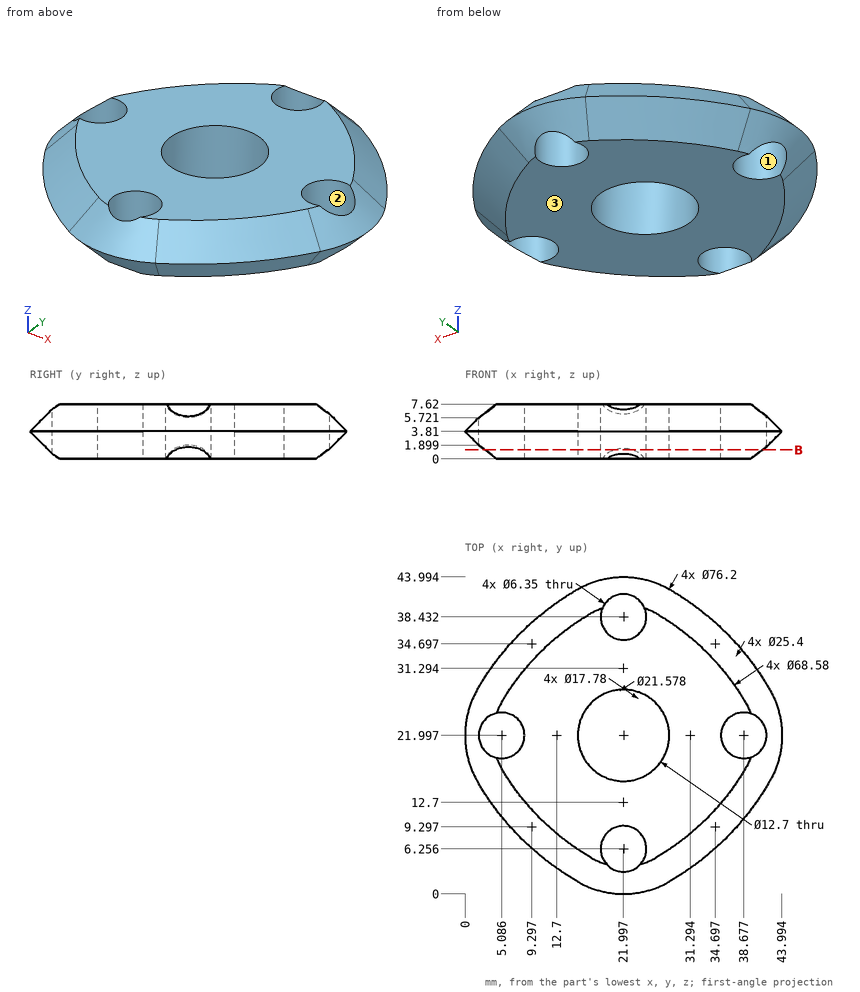
Geometry check sheet. Reference: drawing and pictorial views, mm from the part's lowest x, y, z. Give positions to 0.01 mm unless a question says otherwise; leave off trailing zeros.
1. Go/stop test with flat-tipped pins: pin 1 Ø3 at (y, z) = (8.5, 2.5) entering from +X (1 decimal); pin 2 Ø4 at (y, z) = (32, 2) entering from +X (1 decimal); pin 3 Ø2 at (x, z) = (9, 2) entering from +Y. Record where each tip stops, or that it passes through.
2. Section check B-B, the plane z = 1.25. Count the separate pieces of the cut face and the enclosed holes in it, then the cut area to 3 significant figures.
3. Mould release check, pull along X, two halves, no side actions. Record for the marked faces 1, 2 and 3: released by +X, released by -X, zero draft, split by the parting line, or undercut.
4. Thickness scan on line 1 (Y direction, x = 24, z = 3.5) (1 decimal); line 2 (Y direction, x = 24.5, z = 3) (1 decimal); line 3 (Y direction, x = 18, z = 6) (1 decimal). Record the ranges inside material, lowest first.
Geometry says:
1. pin 1: stops at x = 37.6
1. pin 2: stops at x = 40.5
1. pin 3: stops at y = 36.61
2. separate pieces: 1
2. enclosed holes: 2
2. area: 816 mm2
3. face 1: undercut
3. face 2: undercut
3. face 3: zero draft
4. line 1: y = 0.5 to 3.8, 8.7 to 16, 28 to 36, 40.9 to 43.5
4. line 2: y = 1.1 to 4.3, 8.2 to 16.2, 27.8 to 36.5, 40.4 to 42.9
4. line 3: y = 3 to 17.1, 26.9 to 41
